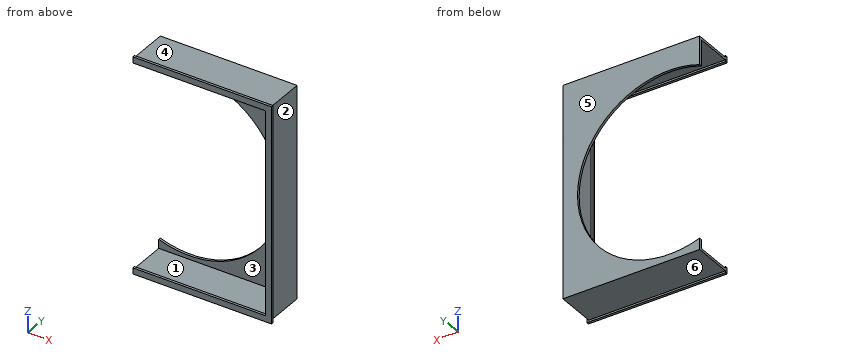
```python
from build123d import *

# Parameters (mm, degrees)
SKETCH_1_W          = 224
SKETCH_1_H          = 174
SKETCH_1_W_2        = 220
SKETCH_1_H_2        = 170
EXTRUDE_1_DEPTH     = 32
SKETCH_2_W          = 227
SKETCH_2_H          = 177
SKETCH_2_W_2        = 217
SKETCH_2_H_2        = 167
EXTRUDE_2_DEPTH     = 2
SKETCH_3_W          = 222
SKETCH_3_H          = 172
SKETCH_3_R          = 75
EXTRUDE_3_DEPTH     = 2
SKETCH_4_W          = 113.5
SKETCH_4_H          = 177
CUT_EXTRUDE_1_DEPTH = 285.974560268


with BuildPart() as part:
    # 草图1 → 凸台-拉伸1 (new body)
    with BuildSketch(Plane(origin=(0, 0, 0), x_dir=(1, 0, 0), z_dir=(0, 1, 0))):
        with Locations((110, -85)):
            Rectangle(SKETCH_1_W, SKETCH_1_H)
        with Locations((110, -85)):
            Rectangle(SKETCH_1_W_2, SKETCH_1_H_2, mode=Mode.SUBTRACT)
    extrude(amount=EXTRUDE_1_DEPTH)

    # 草图2 → 凸台-拉伸2 (add)
    with BuildSketch(Plane(origin=(0, 0, 0), x_dir=(1, 0, 0), z_dir=(0, 1, 0))):
        with Locations((110, -85)):
            Rectangle(SKETCH_2_W, SKETCH_2_H)
        with Locations((110, -85)):
            Rectangle(SKETCH_2_W_2, SKETCH_2_H_2, mode=Mode.SUBTRACT)
    extrude(amount=-EXTRUDE_2_DEPTH)

    # 草图3 → 凸台-拉伸3 (add)
    with BuildSketch(Plane(origin=(0, 32, 0), x_dir=(1, 0, 0), z_dir=(0, 1, 0))):
        with Locations((109, -84)):
            Rectangle(SKETCH_3_W, SKETCH_3_H)
        with Locations(Location((135, -78, 0), (0, 0, 270))):
            Circle(SKETCH_3_R, mode=Mode.SUBTRACT)
    extrude(amount=-EXTRUDE_3_DEPTH)

    # 草图4 → 切除-拉伸1 (cut, through all)
    with BuildSketch(Plane(origin=(0, 32, 0), x_dir=(1, 0, 0), z_dir=(0, 1, 0))):
        with Locations((53.25, -85)):
            Rectangle(SKETCH_4_W, SKETCH_4_H)
    extrude(amount=-CUT_EXTRUDE_1_DEPTH, mode=Mode.SUBTRACT)


solid = part.part
```
Work out the finished part from the listing and answer in its coordinate system (mm). Face numbers are marked on the shaded views. A direction names the side the tool comes from. Coordinates: 2 decimals unless noted, no trailing zeros. Loops run counter-clockwise (first coordinate to the right, second up) from the corner with the lowest first, then second, coordinate; pieces in that order, holes last. Notation, with made-up numbers: (-32.75, 0.5) - (15.25, 0.5) arc R11 ccw to (15.25, 17.5) - close; hole circle Ø10 at (41.5, 34.25). An arc over 180 degrees is marked (long way). Use a Markdown table: item, result.
Item 1: The mould has two halves that part along Z. Classify the marked faces 3, 4, 5 and 6: +Z half, -Z half, draft (parallel to the pull), parting line (faces both ways), or undercut.
Evaluation:
| item | result |
|---|---|
| face 3 | undercut |
| face 4 | +Z half |
| face 5 | draft |
| face 6 | -Z half |
Item 2: Find section A-A, the plane x = 135. Determine the outline of the cut face in (y, z).
Evaluation:
| item | result |
|---|---|
| outline | (-2, -3.5) - (0, -3.5) - (0, -2) - (32, -2) - (32, 3) - (30, 3) - (30, 0) - (0, 0) - (0, 1.5) - (-2, 1.5) - close; (-2, 168.5) - (0, 168.5) - (0, 170) - (30, 170) - (30, 153) - (32, 153) - (32, 172) - (0, 172) - (0, 173.5) - (-2, 173.5) - close |
Item 3: Given pin 1 Ø1.5 at (x, y) = (170.5, 25) entering from +Z; pin 2 Ø2 at (y, z) = (3, 142) entering from +X; pin 3 Ø2 at (y, z) = (-1, 120.5) entering from -X; pin 4 Ø5 at (x, z) = (184.5, 128.5) entering from +Y, each flat-ended and moving along its own axis, determine where each tip first touches the part or whether it passes through.
Evaluation:
| item | result |
|---|---|
| pin 1 | stops at z = 172 |
| pin 2 | stops at x = 222 |
| pin 3 | stops at x = 218.5 |
| pin 4 | passes through |
Item 4: Find section B-B, the plane z = 78. Determine the outline of the cut face in (x, y).
Evaluation:
| item | result |
|---|---|
| outline | (210, 30) - (220, 30) - (220, 0) - (218.5, 0) - (218.5, -2) - (223.5, -2) - (223.5, 0) - (222, 0) - (222, 32) - (210, 32) - close |
Item 5: Find section C-C, the plane y = 8.5. Determine the outline of the cut face in (x, z), and give its area (3 significant figures).
Evaluation:
| item | result |
|---|---|
| outline | (110, -2) - (222, -2) - (222, 172) - (110, 172) - (110, 170) - (220, 170) - (220, 0) - (110, 0) - close |
| area | 788 mm2 |
Item 6: Find section D-D, the plane z = 138. Determine the outline of the cut face in (x, y), and give its area (3 significant figures).
Evaluation:
| item | result |
|---|---|
| outline | (180, 30) - (220, 30) - (220, 0) - (218.5, 0) - (218.5, -2) - (223.5, -2) - (223.5, 0) - (222, 0) - (222, 32) - (180, 32) - close |
| area | 154 mm2 |
Item 7: For the marked faces 1 and 2, determine the directions among +Z, -Z, +X, -X, +Y, -Y from which every point of the face is accessible in a straight line to the end or side of a thin tool.
Evaluation:
| item | result |
|---|---|
| face 1 | -X |
| face 2 | +Z, -Z, +X, +Y |
Item 8: Consider probe 1 along Z at (x, y) = (124, 19.5); probe 2 along Z at (x, y) = (135, 30.6); probe 3 along X at (y, z) = (29.5, 8.5). Determine where each line is inside the solid, lowest interval first. Write a range as from..to.
Evaluation:
| item | result |
|---|---|
| probe 1 | z = -2..0, 170..172 |
| probe 2 | z = -2..3, 153..172 |
| probe 3 | x = 220..222 |
